Could you check a few things on this model? Use its own coordinates, in mm. Face numbers are marked on the shaded views. Coordinates: 2 decimals unless noted, no trailing zeros. Order: outer loops, then holes, each group sorted by start corner. A loop starts at its lowest first (then second) coordinate and runs counter-clockwise, first axis right, second up. Notation, with made-up numbers: (71, -8) -> (97, -8) arc R10 cw to (97, -2) -> close; hole circle Ø3 at (73, -39.75). An arc over 180 degrees is marked (long way). Use a Markdown table: item, result. Add a question column.
1) Thinking about a two-plate mould opening in Y: for the marked faces 1, 2, 3 and 4, which applies, +Y half, -Y half, draft (parallel to the pull), parting line (faces both ways), or undercut?
2) Will these pins go through, and if not, where does the flat tip stop? pin 1 Ø6 at (x, y) = (0, -3) entering from +Z; pin 2 Ø1.5 at (x, z) = (3.5, 5.5) entering from -Y.
3) If I drill on L1, parallel to X at y = 0.5, z = 4.75; L2, parallel to X at y = 2, z = 5.5; L3, parallel to Y at x = 2.75, z = 4.5, over which ranges is the centre line in solid material (lowest first)? Write a range as [from, to].
4) If we section it at C-C (y = 0): Write out the boundary of the cut face in (x, z), plus the area to 3 significant figures.
5) If we section it at D-D (x = 5.25): Write out the boundary of the cut face in (y, z), plus the area to 3 significant figures.
6) If we section it at B-B (x = -2.75): Write out the boundary of the cut face in (y, z), plus the area to 3 significant figures.
7) If we section it at A-A (z = 2.5): Write out the boundary of the cut face in (x, y), plus the area to 3 significant figures.
```python
from build123d import *

# Parameters (mm, degrees)
F0_R     = 4
F1_DEPTH = 6.8


with BuildPart() as f1:
    # F0 (on Top) → F1 (new body)
    with BuildSketch(Plane.XY):
        Polygon((-6.5, 3.7527767497), (-6.5, -3.7527767497), (0, -7.5055534995), (6.5, -3.7527767497), (6.5, 3.7527767497), (0, 7.5055534995), align=None)
        Circle(F0_R, mode=Mode.SUBTRACT)
    extrude(amount=F1_DEPTH)

    # F2 (on Right) → F3 (revolve, cut)
    with BuildSketch(Plane.YZ):
        Polygon((7.0055534995, 0), (7.5055534995, 0), (7.5055534995, 0.5), align=None)
    revolve(axis=Axis((0, 0, 0), (0, 0, -1)), mode=Mode.SUBTRACT)


solid = f1.part
```
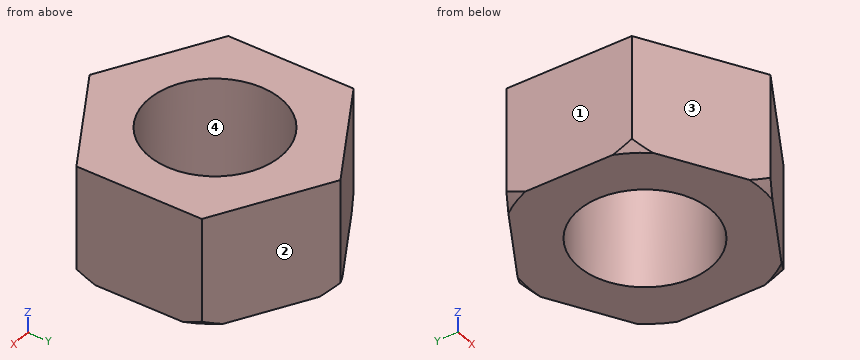
Answer sheet:
| question | item | result |
|---|---|---|
| 1 | face 1 | draft |
| 1 | face 2 | +Y half |
| 1 | face 3 | -Y half |
| 1 | face 4 | undercut |
| 2 | pin 1 | z = 6.8 |
| 2 | pin 2 | y = -5.92 |
| 3 | L1 | [-6.5, -3.97], [3.97, 6.5] |
| 3 | L2 | [-6.5, -3.46], [3.46, 6.5] |
| 3 | L3 | [-5.92, -2.9], [2.9, 5.92] |
| 4 | outline | (-6.5, 0) -> (-4, 0) -> (-4, 6.8) -> (-6.5, 6.8) -> close; (4, 0) -> (6.5, 0) -> (6.5, 6.8) -> (4, 6.8) -> close |
| 4 | area | 34.0 mm2 |
| 5 | outline | (-4.47, 0) -> (4.47, 0) -> (4.47, 6.8) -> (-4.47, 6.8) -> close |
| 5 | area | 60.9 mm2 |
| 6 | outline | (-5.92, 0) -> (-2.9, 0) -> (-2.9, 6.8) -> (-5.92, 6.8) -> close; (2.9, 0) -> (5.92, 0) -> (5.92, 6.8) -> (2.9, 6.8) -> close |
| 6 | area | 41.0 mm2 |
| 7 | outline | (-6.5, -3.75) -> (0, -7.51) -> (6.5, -3.75) -> (6.5, 3.75) -> (0, 7.51) -> (-6.5, 3.75) -> close; hole circle Ø8 at (0, 0) |
| 7 | area | 96.1 mm2 |
